from build123d import *


with BuildPart() as f3:
    # F0 (on Front) → F3 section 0
    with BuildSketch(Plane.XZ, mode=Mode.PRIVATE) as f3_s0:
        Polygon((0, 54.938529), (-32.991804, 24.241803), (-69.713116, -6.168033), (-25.819672, -22.807376), (-49.344264, -59.815578), (5.163935, -46.331968), (64.83607, -60.389347), (30.983604, -18.217213), (72.868854, 11.331968), (27.801723, 25.058175), align=None)
    loft([f3_s0.sketch, Vertex(0, -100, -4.188326)])


solid = f3.part
Geometry: final body of the model. Coordinates: model frame, mm. A direction names the side the tool comes from. Coordinates: 2 decimals unless noted, no trailing zeros. Write each loop counter-clockwise with the first axis right and the second up, starting at its lowest first coordinate (ties: lowest second). Pieces come first, ordered by that corner, then holes. Notation, with made-up numbers: (-25.5, -19) - (6.5, -19) arc R31 ccw to (6.5, 11) - close; hole circle Ø6 at (-5.75, 51.5). An arc over 180 degrees is marked (long way). Return JSON: item names as keys, results as strings.
Item 1: Section query B-B (y = -48.5). Output: boundary loops of the cut face in (x, z).
Completed:
{"outline": "(-35.9, -5.21) - (-13.3, -13.78) - (-25.41, -32.84) - (2.66, -25.89) - (33.39, -33.13) - (15.96, -11.41) - (37.53, 3.8) - (14.32, 10.87) - (0, 26.26) - (-16.99, 10.45) - close"}
Item 2: Pin query (flat end, axial travel): pin 1 Ø12 at (x, y) = (35.5, -60.5) entering from +Z; pin 2 Ø1 at (x, y) = (37, -52.5) entering from +Z; pin 3 Ø1 at (y, z) = (-43, -33.5) entering from +X; pin 4 Ø3 at (y, z) = (-59.5, -1.5) entering from +X. Return the tip coordinate at first contact, or that it passes through.
Completed:
{"pin 1": "stops at z = 2.81", "pin 2": "passes through", "pin 3": "stops at x = 35.18", "pin 4": "stops at x = 26.67"}
Item 3: Section query A-A (x = 43). Output: boundary loops of the cut face in (y, z), and give its area (3 significant figures).
Completed:
{"outline": "(-40.99, 4.97) - (0, -9.74) - (0, 20.43) - close; (-33.68, -41.46) - (0, -55.25) - (0, -33.19) - close", "area": "990 mm2"}
Item 4: Section query C-C (z = -16.5). Output: boundary loops of the cut face in (x, y), and give its area (3 significant figures).
Completed:
{"outline": "(-42.46, 0) - (-17.07, -33.88) - (-10.92, -77.87) - (1.51, -70.79) - (14.2, -78.09) - (27.19, -12.24) - (33.42, 0) - close", "area": "3,270 mm2"}
Item 5: Section query D-D (x = -17). Output: boundary loops of the cut face in (y, z).
Completed:
{"outline": "(-75.61, -4.67) - (-34.16, -16.45) - (-65.55, -23.35) - (0, -51.81) - (0, 39.12) - (-48.47, 10.46) - close"}
Item 6: Line query: L1, parallel to Z at x = -8, y = -71.5; L2, parallel to X at y = -11, z = -23; L3, parallel to Z at x = 25, y = -36. Output: solid intervals per line, ascending.
Completed:
{"L1": "z = -18.54 to -10.5, -9.25 to 5.22", "L2": "x = -24.4 to 32.65", "L3": "z = -36.27 to -19.61, -9.52 to 12.33"}
Item 7: Reachability of faces 1 (the face through (19.62, -31.71, -36.76)), 2 (the face through (32.55, -35.42, -4.4)), 3 (the face through (-11.53, -28.48, 27.37)), 4 (the face through (-24.94, -31.71, -28.4)) from +Z, -Z, +X, -X, +Y, -Y: full face, straight path, thin tool, end or side. Return the list, or none.
Completed:
{"face 1": "-Z, -Y", "face 2": "+X, -Y", "face 3": "+Z, -X, -Y", "face 4": "-X, -Y"}
Item 8: Pull-direction query (Z, two-part tool) for faces 5 (the face through (-32.25, -31.71, -11.36)), 6 (the face through (-1, 0, -4)), 7 (the face through (-9.695, -28.478, -37.642)); classes: +Z half, -Z half, draft (parallel to the pull), parting line (faces both ways), or undercut.
Completed:
{"face 5": "undercut", "face 6": "draft", "face 7": "-Z half"}
